from build123d import *

# Parameters (mm, degrees)
EXTRUDE_2_DEPTH = 6


with BuildPart() as part:
    # Эскиз1 → Бобышка-Вытянуть2 (new body)
    with BuildSketch(Plane(origin=(0, 0, 0), x_dir=(0, 0, -1), z_dir=(1, 0, 0))):
        Polygon((240, -90), (-240, -90), (-240, -70), (-250, -70), (-250, -20), (-240, -20), (-240, 20), (-250, 20), (-250, 70), (-240, 70), (-240, 88.6), (-198.210576245, 88.6), (-198.210576245, 83.6), (-188.210576245, 83.6), (-188.210576245, 88.6), (-153.210576245, 88.6), (-153.210576245, 83.6), (-143.210576245, 83.6), (-143.210576245, 88.6), (-108.210576245, 88.6), (-108.210576245, 83.6), (-98.210576245, 83.6), (-98.210576245, 88.6), (-63.210576245, 88.6), (-63.210576245, 83.6), (-53.210576245, 83.6), (-53.210576245, 88.6), (-18.210576245, 88.6), (-18.210576245, 83.6), (-8.210576245, 83.6), (-8.210576245, 88.6), (26.789423755, 88.6), (26.789423755, 83.6), (36.789423755, 83.6), (36.789423755, 88.6), (71.789423755, 88.6), (71.789423755, 83.6), (81.789423755, 83.6), (81.789423755, 88.6), (116.789423755, 88.6), (116.789423755, 83.6), (126.789423755, 83.6), (126.789423755, 88.6), (161.789423755, 88.6), (161.789423755, 83.6), (171.789423755, 83.6), (171.789423755, 88.6), (240, 88.6), (240, 70), (250, 70), (250, 20), (240, 20), (240, -20), (250, -20), (250, -70), (240, -70), align=None)
    extrude(amount=EXTRUDE_2_DEPTH)


solid = part.part
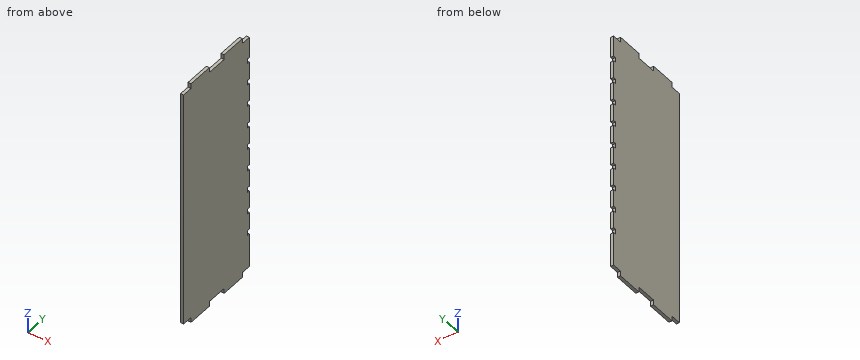
The model under review builds one solid part; all positions refer to its coordinate system, in mm. Round coordinates to 2 decimals unless told otherwise and drop trailing zeros. Write each loop counter-clockwise with the first axis right and the second up, starting at its lowest first coordinate (ties: lowest second). Pieces come first, ordered by that corner, then holes. Notation, with made-up numbers: (57, 76.25) -> (69, 76.25) arc R32 cw to (69, 104.25) -> close; hole circle Ø10 at (2, 63). An arc over 180 degrees is marked (long way). Answer as a JSON object with one key per item and string values.
1. We need section A-A on y = -79. State the section outline as (x, z) points, and give its area (3 significant figures).
Results found:
{"outline": "(0, -240) -> (6, -240) -> (6, 240) -> (0, 240) -> close", "area": "2,880 mm^2"}
2. To check wall thickness, follow line 1 along Z through (x, y) = (2.6, -17); line 2 along Y through (x, z) = (5.1, 108). State the ranges of each line that lie inside material, in increasing order.
Results found:
{"line 1": "z = -240 to 240", "line 2": "y = -90 to 83.6"}
3. Clearance check with flat-ended pins moving along their axes: pin 1 (2.5 mm diameter, centred on x = 3, y = 87, fed in from +Z); pin 2 (1.8 mm diameter, centred on x = 3.5, z = -31, fed in from +Y); pin 3 (1.5 mm diameter, centred on x = 4.5, y = -15.5, fed in from -Z); pin 4 (1.5 mm diameter, centred on y = -59.5, z = 19.5, fed in from -X). State where each tip first meets the part, or that it passes through.
Results found:
{"pin 1": "stops at z = 240", "pin 2": "stops at y = 83.6", "pin 3": "stops at z = -240", "pin 4": "stops at x = 0"}
